Could you check a few things on this model? Use its own coordinates, in mm. Round coordinates to 2 decimals unless told otherwise and drop trailing zeros. Write each loop counter-clockwise with the first axis right and the second up, starting at its lowest first coordinate (ties: lowest second). Pieces come first, ordered by that corner, then holes. Notation, with made-up numbers: (48, 1) -> (94, 1) arc R23 ccw to (94, 27) -> close; hole circle Ø1 at (35.5, 75.25). An arc over 180 degrees is marked (long way). Answer in a Markdown table with one row per item.
from build123d import *

# Parameters (mm, degrees)
F1_DEPTH  = 6.35
F3_DEPTH  = 279.4
F4_W      = 101.6
F4_H      = 3.175
F5_DEPTH  = 3.175
F6_W      = 12.7
F6_H      = 4.1792877018
F7_DEPTH  = 25.4
F8_W      = 101.6
F8_H      = 6.35
F9_DEPTH  = 25.4
F11_DEPTH = 69.851
F12_W     = 6.2937450767
F12_H     = 5.9905603992
F13_DEPTH = 6.35
F14_W     = 6.4354827628
F14_H     = 1.8108228737
F15_DEPTH = 25.4
F16_W     = 6.3454108313
F16_H     = 1.71593274
F17_DEPTH = 25.4


# Not quite as in the source:
# - a feature names something its author has since deleted; it is built from what else it names


with BuildPart() as f1:
    # F0 (on Front) → F1 (new body, symmetric)
    with BuildSketch(Plane.XZ):
        Polygon((0, 38.1), (0, 0), (101.6, 0), (101.6, 76.2), (0, 76.2), align=None)
    extrude(amount=F1_DEPTH, both=True)

    # F2 (on face) → F3 (cut)
    with BuildSketch(Plane(origin=(0, 0, 0), x_dir=(0, -1, 0), z_dir=(-1, 0, 0))):
        Polygon((0, 45.9105), (0, 38.1), (6.35, 39.9208331996), (6.35, 44.0896668004), align=None)
    extrude(amount=-F3_DEPTH, mode=Mode.SUBTRACT)

    # F4 (on face) → F5 (cut)
    with BuildSketch(Plane(origin=(0, 6.35, 0), x_dir=(-1, 0, 0), z_dir=(0, 1, 0))):
        with Locations((-50.8, 4.7625)):
            Rectangle(F4_W, F4_H)
    extrude(amount=-F5_DEPTH, mode=Mode.SUBTRACT)

    # F6 (on face) → F7 (cut)
    with BuildSketch(Plane.XZ):
        with BuildLine():
            Line((50.8, 39.8820452392), (50.8, 44.0613329411))
            ThreePointArc((50.8, 44.0613329411), (48.7103561491, 41.9716890901), (50.8, 39.8820452392))
        make_face()
        with Locations((57.15, 41.9716890901)):
            Rectangle(F6_W, F6_H)
        with BuildLine():
            ThreePointArc((63.5, 39.8820452392), (65.5896438509, 41.9716890901), (63.5, 44.0613329411))
            Line((63.5, 44.0613329411), (63.5, 39.8820452392))
        make_face()
    extrude(amount=-F7_DEPTH, mode=Mode.SUBTRACT)

    # F8 (on face) → F9 (cut)
    with BuildSketch(Plane.XZ.offset(6.35)):
        with Locations((50.8, 73.025)):
            Rectangle(F8_W, F8_H)
    extrude(amount=-F9_DEPTH, mode=Mode.SUBTRACT)

    # F10 (on face) → F11 (cut, through all)
    with BuildSketch(Plane.XY.offset(69.85)):
        Polygon((0, 6.35), (0, -6.35), (12.7, 6.35), align=None)
        Polygon((88.9, 6.35), (101.6, -6.35), (101.6, 6.35), align=None)
    extrude(amount=-F11_DEPTH, mode=Mode.SUBTRACT)

    # F12 (on face) → F13 (cut)
    with BuildSketch(Plane.XZ.offset(6.35)):
        with Locations((98.4531274617, 41.0943866008)):
            Rectangle(F12_W, F12_H)
        Polygon((101.6, 45.8681471646), (95.3062549233, 45.9736101329), (95.3062549233, 44.0896668004), (101.6, 44.0896668004), align=None)
    extrude(amount=-F13_DEPTH, mode=Mode.SUBTRACT)

    # F14 (on face) → F15 (cut)
    with BuildSketch(Plane.XZ.offset(6.35)):
        with Locations((3.2177413814, 39.0154217627)):
            Rectangle(F14_W, F14_H)
    extrude(amount=-F15_DEPTH, mode=Mode.SUBTRACT)

    # F16 (on face) → F17 (cut)
    with BuildSketch(Plane.XZ.offset(6.35)):
        with Locations((3.1727054156, 44.9476331705)):
            Rectangle(F16_W, F16_H)
    extrude(amount=-F17_DEPTH, mode=Mode.SUBTRACT)


solid = f1.part
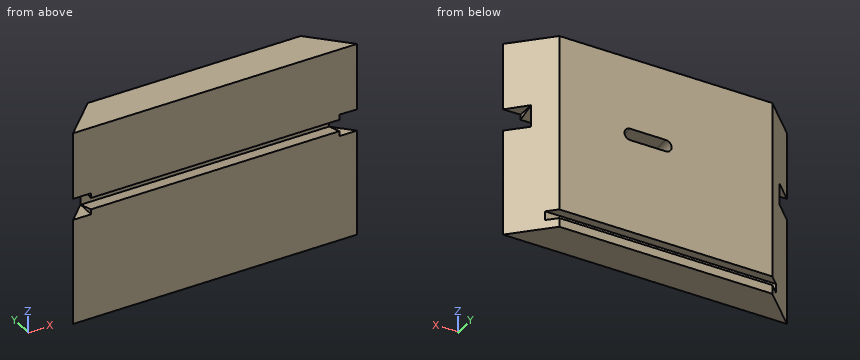
1) Imagine slicing it at B-B, the plane z = 43. Please give me the cut outline in (x, y), plus the area to 3 significant figures.
Findings:
| item | result |
|---|---|
| outline | (6.35, 0) -> (48.98, 0) -> (48.98, 6.35) -> (12.7, 6.35) -> close; (65.32, 0) -> (95.25, 0) -> (88.9, 6.35) -> (65.32, 6.35) -> close |
| area | 420 mm^2 |
2) Please list where these lines run through material, in increasing order: line 1 (Z direction, x = 35, y = 5.75) (3 decimals); line 2 (Y direction, x = 6, z = 16.5); line 3 (Z direction, x = 97, y = -5).
Findings:
| item | result |
|---|---|
| line 1 | z = 0 to 3.175, 6.35 to 69.85 |
| line 2 | y = -6.35 to -0.35 |
| line 3 | z = 0 to 38.1, 45.95 to 69.85 |
3) Imagine slicing it at C-C, the plane z = 19.5. Please give me the cut outline in (x, y), plus the area to 3 significant figures.
Findings:
| item | result |
|---|---|
| outline | (0, -6.35) -> (101.6, -6.35) -> (88.9, 6.35) -> (12.7, 6.35) -> close |
| area | 1,130 mm^2 |
4) Imagine slicing it at A-A, the plane y = 5.25. Please give me the cut outline in (x, z) (3 decimals), plus the area to 3 significant figures.
Findings:
| item | result |
|---|---|
| outline | (11.6, 0) -> (90, 0) -> (90, 3.175) -> (11.6, 3.175) -> close; (11.6, 6.35) -> (90, 6.35) -> (90, 69.85) -> (11.6, 69.85) -> close; hole (50.8, 39.882) -> (63.5, 39.882) arc R2.09 ccw to (63.5, 44.061) -> (50.8, 44.061) arc R2.09 ccw to start |
| area | 5,160 mm^2 |
5) For pin 1 (1.4 mm diameter, centred on y = -4.5, z = 45.5, fed in from -X); pin 2 (2 mm diameter, centred on y = -2.5, z = 45.5, fed in from +X); pin 3 (1.5 mm diameter, centred on y = 2.5, z = 23.5, fed in from -X); pin 4 (1.9 mm diameter, centred on x = 99, y = -1.5, fed in from +Z) (3 decimals), each with a flat end and sliding along its axis, tell me the tip position at first contact or that it passes through.
Findings:
| item | result |
|---|---|
| pin 1 | stops at x = 1.22 |
| pin 2 | stops at x = 98.66 |
| pin 3 | stops at x = 8.1 |
| pin 4 | passes through |
